Check sheet for the drawn part. Datum: minimum x, y, z corner. Units: mm. A direction names the side the tool comes from. Give positions to 0.01 mm unless a question says otherwise; leave off trailing zeros. Loops run counter-clockwise (first coordinate to the right, second up) from the corner with the lowest first, then second, coordinate; pieces in that order, holes last.
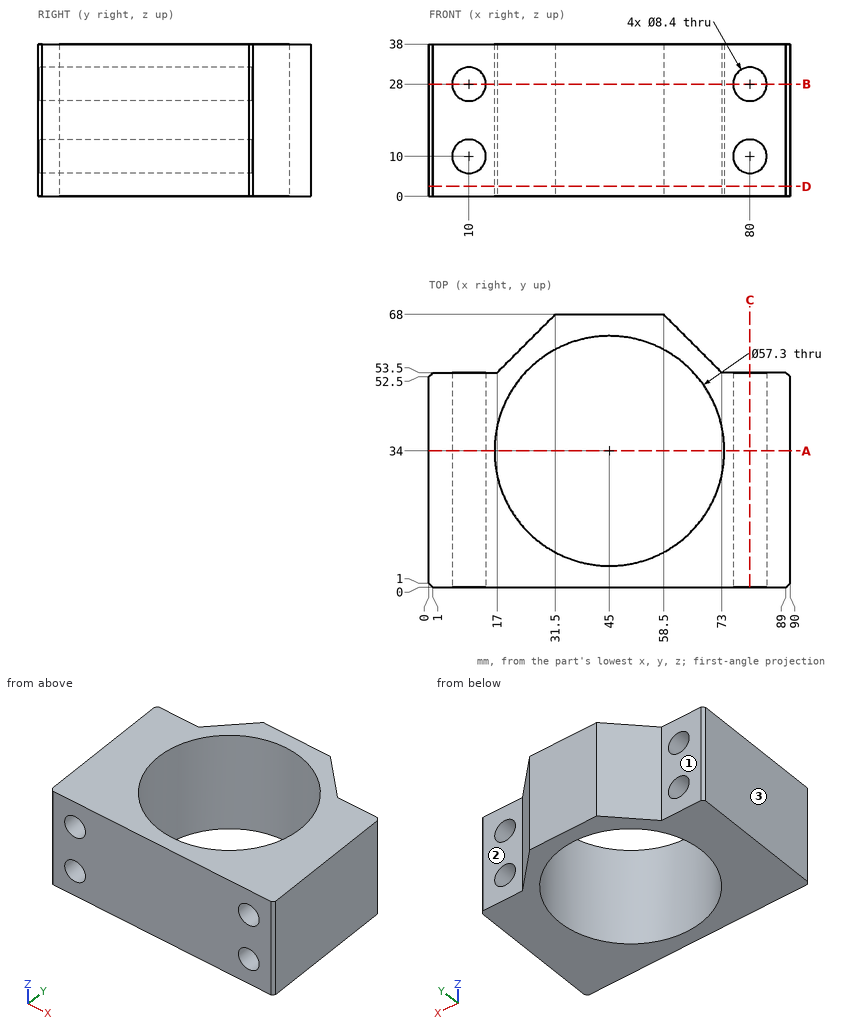
(1) Gauge pin test, flat ends, axial feed: pin 1 Ø10 at (x, z) = (13, 29.5) entering from -Y; pin 2 Ø2 at (x, z) = (20.5, 20) entering from +Y; pin 3 Ø13.5 at (x, z) = (80, 10) entering from +Y; pin 4 Ø4 at (x, z) = (23.5, 5.5) entering from +Y. Record the tip position at first contact, or that the pin passes through.
(2) Section check A-A on y = 34. Record the boundary of the cut face in (x, z), plus the area to 3 significant figures.
(3) Section check D-D on z = 2.5. Record the boundary of the cut face in (x, y).
(4) Section check C-C on x = 80. Record the boundary of the cut face in (y, z).
(5) Access from +Z, -Z, +X, -X, +Y, -Y to the whole of each face (thin tool, end or side, straight path). Record for the marked faces 1, 2 and 3.
(6) Material ranges on line 1 (Z direction, x = 10, y = 38); line 2 (X direction, y = 36, z = 31); line 3 (X direction, y = 22, z = 31), recorded low to high.
(7) Section check B-B on z = 28. Record the boundary of the cut face in (x, y).
Computed values:
1. pin 1: stops at y = 0
1. pin 2: stops at y = 58
1. pin 3: stops at y = 53.5
1. pin 4: stops at y = 62
2. outline: (0, 0) - (16.35, 0) - (16.35, 38) - (0, 38) - close; (73.65, 0) - (90, 0) - (90, 38) - (73.65, 38) - close; hole circle Ø8.4 at (10, 10); hole circle Ø8.4 at (10, 28); hole circle Ø8.4 at (80, 10); hole circle Ø8.4 at (80, 28)
2. area: 1,020 mm2
3. outline: (0, 1) - (1, 0) - (89, 0) - (90, 1) - (90, 52.5) - (89, 53.5) - (73, 53.5) - (58.5, 68) - (31.5, 68) - (17, 53.5) - (1, 53.5) - (0, 52.5) - close; hole circle Ø57.3 at (45, 34)
4. outline: (0, 0) - (53.5, 0) - (53.5, 5.8) - (0, 5.8) - close; (0, 14.2) - (53.5, 14.2) - (53.5, 23.8) - (0, 23.8) - close; (0, 32.2) - (53.5, 32.2) - (53.5, 38) - (0, 38) - close
5. face 1: +Z, -Z, -X, +Y
5. face 2: +Z, -Z, +X, +Y
5. face 3: +Z, -Z, -X, +Y, -Y
6. line 1: z = 0 to 5.8, 14.2 to 23.8, 32.2 to 38
6. line 2: x = 0 to 7.06, 12.94 to 16.42, 73.58 to 77.06, 82.94 to 90
6. line 3: x = 0 to 7.06, 12.94 to 18.98, 71.02 to 77.06, 82.94 to 90
7. outline: (0, 1) - (1, 0) - (5.8, 0) - (5.8, 53.5) - (1, 53.5) - (0, 52.5) - close; (14.2, 0) - (75.8, 0) - (75.8, 53.5) - (73, 53.5) - (58.5, 68) - (31.5, 68) - (17, 53.5) - (14.2, 53.5) - close; (84.2, 0) - (89, 0) - (90, 1) - (90, 52.5) - (89, 53.5) - (84.2, 53.5) - close; hole circle Ø57.3 at (45, 34)
